from build123d import *

# Parameters (mm, degrees)
SKETCH1_W           = 82.55
SKETCH1_H           = 127.0659892
SKETCH1_R           = 5.08
SKETCH1_R_2         = 1.27
BASE_EXTRUDE_DEPTH  = 2.54
SKETCH7_R           = 2.55
BOSS_EXTRUDE6_DEPTH = 27.686
SKETCH7_3_R         = 3.81
BOSS_EXTRUDE7_DEPTH = 12.192
CHAMFER1_SIZE       = 0.63
CHAMFER2_SIZE       = 0.63
CHAMFER3_SIZE       = 0.63
CHAMFER4_SIZE       = 0.63
SKETCH8_W           = 23.876
SKETCH8_H           = 41.25
CUT_EXTRUDE1_DEPTH  = 10


with BuildPart() as part:
    # Sketch1 → base extrude (new body)
    with BuildSketch(Plane(origin=(0, 0, 0), x_dir=(1, 0, 0), z_dir=(0, 1, 0))):
        with Locations((41.275, -100.8050054)):
            Rectangle(SKETCH1_W, SKETCH1_H)
        with Locations(Location((41.275, -58.1000108, 0), (0, 0, 270))):
            Circle(SKETCH1_R, mode=Mode.SUBTRACT)
        with Locations(Location((25.527, -42.3520108, 0), (0, 0, 270))):
            Circle(SKETCH1_R_2, mode=Mode.SUBTRACT)
        with Locations(Location((57.023, -42.3520108, 0), (0, 0, 270))):
            Circle(SKETCH1_R_2, mode=Mode.SUBTRACT)
        with Locations(Location((57.023, -73.8480108, 0), (0, 0, 270))):
            Circle(SKETCH1_R_2, mode=Mode.SUBTRACT)
        with Locations(Location((25.527, -73.8480108, 0), (0, 0, 270))):
            Circle(SKETCH1_R_2, mode=Mode.SUBTRACT)
    extrude(amount=BASE_EXTRUDE_DEPTH)

    # Sketch7 → Boss-Extrude6 (add)
    with BuildSketch(Plane(origin=(0, 2.54, 0), x_dir=(1, 0, 0), z_dir=(0, 1, 0))):
        with Locations(Location((65.151, -102.529, 0), (0, 0, 270))):
            Circle(SKETCH7_R)
        with Locations(Location((17.399, -102.529, 0), (0, 0, 270))):
            Circle(SKETCH7_R)
        with Locations(Location((65.151, -143.779, 0), (0, 0, 270))):
            Circle(SKETCH7_R)
        with Locations(Location((17.399, -143.779, 0), (0, 0, 270))):
            Circle(SKETCH7_R)
    extrude(amount=BOSS_EXTRUDE6_DEPTH)

    # Sketch7<3> → Boss-Extrude7 (add)
    with BuildSketch(Plane(origin=(0, 2.54, 0), x_dir=(1, 0, 0), z_dir=(0, 1, 0))):
        with Locations(Location((65.151, -102.529, 0), (0, 0, 90))):
            Circle(SKETCH7_3_R)
        with Locations(Location((17.399, -102.529, 0), (0, 0, 90))):
            Circle(SKETCH7_3_R)
        with Locations(Location((65.151, -143.779, 0), (0, 0, 90))):
            Circle(SKETCH7_3_R)
        with Locations(Location((17.399, -143.779, 0), (0, 0, 90))):
            Circle(SKETCH7_3_R)
    extrude(amount=BOSS_EXTRUDE7_DEPTH)

    # Chamfer1
    chamfer1_edges = [part.edges().sort_by_distance(p)[0] for p in [
        (65.151, 14.732, 99.979),
        (65.151, 2.54, 106.339),
        (65.151, 14.732, 106.339),
    ]]
    chamfer(chamfer1_edges, length=CHAMFER1_SIZE - 0.0001)  # a hair under: the kernel refuses the full size

    # Chamfer2
    chamfer2_edges = [part.edges().sort_by_distance(p)[0] for p in [
        (17.399, 14.732, 99.979),
        (17.399, 2.54, 106.339),
        (17.399, 14.732, 106.339),
    ]]
    chamfer(chamfer2_edges, length=CHAMFER2_SIZE - 0.0001)  # a hair under: the kernel refuses the full size

    # Chamfer3
    chamfer3_edges = [part.edges().sort_by_distance(p)[0] for p in [
        (65.151, 14.732, 141.229),
        (65.151, 2.54, 147.589),
        (65.151, 14.732, 147.589),
    ]]
    chamfer(chamfer3_edges, length=CHAMFER3_SIZE - 0.0001)  # a hair under: the kernel refuses the full size

    # Chamfer4
    chamfer4_edges = [part.edges().sort_by_distance(p)[0] for p in [
        (17.399, 14.732, 141.229),
        (17.399, 2.54, 147.589),
        (17.399, 14.732, 147.589),
    ]]
    chamfer(chamfer4_edges, length=CHAMFER4_SIZE - 0.0001)  # a hair under: the kernel refuses the full size

    # Sketch8 → Cut-Extrude1 (cut)
    with BuildSketch(Plane(origin=(0, 2.54, 0), x_dir=(1, 0, 0), z_dir=(0, 1, 0))):
        Polygon((82.55, -37.2720108), (61.9125, -37.2720108), (75.670833333, -121.982670267), (73.536197868, -148.268757917), (41.275, -164.338), (82.55, -164.338), align=None)
        Polygon((6.879166667, -121.982670267), (20.6375, -37.2720108), (0, -37.2720108), (0, -164.338), (41.275, -164.338), (9.013802132, -148.268757917), align=None)
        with Locations((41.275, -123.154)):
            Rectangle(SKETCH8_W, SKETCH8_H)
    extrude(amount=-CUT_EXTRUDE1_DEPTH, mode=Mode.SUBTRACT)


solid = part.part
Build history of the part. All positions in model axes, mm. A direction names the side the tool comes from. Round coordinates to 2 decimals unless told otherwise and drop trailing zeros. Write each loop counter-clockwise with the first axis right and the second up, starting at its lowest first coordinate (ties: lowest second). Pieces come first, ordered by that corner, then holes. Notation, with made-up numbers: M 69,32 L 87,32 A13 cw 87,37 Z; hole C 72,70 d1. An arc over 180 degrees is marked long. Answer in a Markdown table with one row per item.
1. Flat gauge pins, fed straight in: P1, Ø2, axis at x = 45.5, y = 1.5, coming from the +Z side; P2, Ø4, axis at x = 56, z = 103.5, coming from the -Y side; P3, Ø20.5, axis at x = 49.5, z = 77, coming from the +Y side; P4, Ø1.3, axis at y = 1, z = 118.5, coming from the +X side. Where does each tip first touch, or does it go through?
Geometry check:
| item | result |
|---|---|
| P1 | z = 162.73 |
| P2 | y = 0 |
| P3 | y = 2.54 |
| P4 | x = 75.21 |
2. Mould opens along X. For faces 1 (the face through (53.213, 1, 123)), 2 (the face through (24.287, 1.252, 42.077)), 3 (the face through (17, 30.226, 144)), 4 (the face through (74.62, 1.29, 134.94)) say: +X half, -X half, draft (parallel to the pull), parting line (faces both ways), or undercut.
Geometry check:
| item | result |
|---|---|
| face 1 | undercut |
| face 2 | undercut |
| face 3 | draft |
| face 4 | +X half |
3. Saw through at C-C (z = 54.5). List the corners of the cut face in (x, y).
Geometry check:
| item | result |
|---|---|
| outline | M 17.84,0 L 37.69,0 L 37.69,2.54 L 17.84,2.54 Z; M 44.86,0 L 64.71,0 L 64.71,2.54 L 44.86,2.54 Z |
4. Probe L1, parallel to Y at x = 32, z = 78.5; L2, parallel to X at y = 7, z = 141; L3, parallel to Z at x = 64.5, y = 13.5. List the from-to ranges inside material, lowest first. Write a range as [from, to].
Geometry check:
| item | result |
|---|---|
| L1 | [0, 2.54] |
| L2 | [14.79, 20.01], [62.54, 67.76] |
| L3 | [98.78, 106.28], [140.03, 147.53] |
5. Which spindle directions (+Z, -Z, +X, -X, +Y, -Y) get a long thin tool onto all of the face, cutting with end or side? Do faces 5 (the face through (41, 1, 143.779)), 6 (the face through (7.96, 1.29, 135.31)), 7 (the face through (64.174, 22.69, 104.885)). Say none if no direction does.
Geometry check:
| item | result |
|---|---|
| face 5 | +Y, -Y |
| face 6 | +Z, -X, +Y, -Y |
| face 7 | +Y |
6. Saw through at A-A (z = 135). List the corners of the cut face in (x, y), and give its area (3 significant figures).
Geometry check:
| item | result |
|---|---|
| outline | M 7.94,0 L 29.34,0 L 29.34,2.54 L 7.94,2.54 Z; M 53.21,0 L 74.61,0 L 74.61,2.54 L 53.21,2.54 Z |
| area | 109 mm2 |
7. Saw through at D-D (x = 71). List the corners of the cut face in (y, z).
Geometry check:
| item | result |
|---|---|
| outline | M 0,93.22 L 2.54,93.22 L 2.54,149.53 L 0,149.53 Z |
8. Saw through at B-B (y = 12). List the corners of the cut face in (x, z), and give its area (3 significant figures).
Geometry check:
| item | result |
|---|---|
| outline | C 17.4,102.53 d7.62; C 17.4,143.78 d7.62; C 65.15,102.53 d7.62; C 65.15,143.78 d7.62 |
| area | 182 mm2 |
